from build123d import *

# Parameters (mm, degrees)
SKETCH_1_R      = 13
SKETCH_1_R_2    = 2
SKETCH_1_R_3    = 1.5
EXTRUDE_1_DEPTH = 3
FILLET_1_R      = 2


with BuildPart() as part:
    # 草图1 → 凸台-拉伸1 (new body)
    with BuildSketch(Plane.XY):
        with BuildLine():
            Line((0, 21), (32.5, 21))
            Line((32.5, 21), (32.5, 5))
            Line((32.5, 5), (47.5, 5))
            Line((47.5, 5), (47.5, 8))
            ThreePointArc((47.5, 8), (49, 9.5), (50.5, 8))
            Line((50.5, 8), (50.5, -21))
            Line((50.5, -21), (0, -21))
            ThreePointArc((0, -21), (-21, 0), (0, 21))
        make_face()
        Circle(SKETCH_1_R, mode=Mode.SUBTRACT)
        with Locations((17.5, 0)):
            Circle(SKETCH_1_R_2, mode=Mode.SUBTRACT)
        with Locations((0, -17.5)):
            Circle(SKETCH_1_R_2, mode=Mode.SUBTRACT)
        with Locations((-17.5, 0)):
            Circle(SKETCH_1_R_2, mode=Mode.SUBTRACT)
        with Locations((0, 17.5)):
            Circle(SKETCH_1_R_2, mode=Mode.SUBTRACT)
        with Locations((40, -7.5)):
            Circle(SKETCH_1_R_3, mode=Mode.SUBTRACT)
        with Locations((40, -17.5)):
            Circle(SKETCH_1_R_3, mode=Mode.SUBTRACT)
        with Locations((24.5, 15)):
            Circle(SKETCH_1_R_3, mode=Mode.SUBTRACT)
        with Locations((24.5, -15)):
            Circle(SKETCH_1_R_3, mode=Mode.SUBTRACT)
    extrude(amount=EXTRUDE_1_DEPTH)

    # 圆角1
    fillet_1_edges = [part.edges().sort_by_distance(p)[0] for p in [
        (32.5, 21, 1.5),
        (50.5, -21, 1.5),
    ]]
    fillet(fillet_1_edges, radius=FILLET_1_R)


solid = part.part
Input: part model. Units: mm. Frame: model coordinates. A direction names the side the tool comes from. Coordinates: 2 decimals unless noted, no trailing zeros. Loops run counter-clockwise (first coordinate to the right, second up) from the corner with the lowest first, then second, coordinate; pieces in that order, holes last. Notation, with made-up numbers: (85, 29) -> (144, 29) arc R16 ccw to (144, 36) -> close; hole circle Ø1 at (59.5, -18.75). An arc over 180 degrees is marked (long way). Write each question's results on one line, items separated by ' | '. Start each with the question number.
Q1. Section D-D, the plane x = -6. Return the cut outline in (y, z), plus the area to 3 significant figures.
Q2. Section C-C, the plane y = 11. Return the cut outline in (x, z).
Q3. Section B-B, the plane z = 2.5. State how many separate pieces and enclosed holes the cut face has, plus the area to 3 significant figures.
Q4. Reachability of faces 1 (the flat face through (32.5, 12, 1)), 2 (the flat face through (50.5, -5, 1)) from +Z, -Z, +X, -X, +Y, -Y: full face, straight path, thin tool, end or side. Return the list, or none.
Q5. Pin query (flat end, axial travel): pin 1 (0.9 mm diameter, centred on x = 40.5, z = 2, fed in from +Y); pin 2 (3 mm diameter, centred on x = 0, y = 17.5, fed in from +Z); pin 3 (1 mm diameter, centred on x = -8, z = 0.5, fed in from -Y). Return the tip coordinate at first contact, or that it passes through.
Q6. Section A-A, the plane x = 40. Return the cut outline in (y, z).
Q7. Ray query, line 1 (Y direction, x = 24.5, z = 1.6); line 2 (X direction, y = -18, z = 1.8); line 3 (X direction, y = 7, z = 0.6). Return the intervals inside material, ascending. Write a range as from..to.
Q8. Pull-direction query (Y, two-part tool) for faces 3 (the flat face through (40, 5, 1)), 4 (the flat face through (23, 0, 0)), 5 (the cylindrical face through (-19.1, -1.2, 1.5)); classes: released by +Y, released by -Y, zero draft, split by the parting line, or undercut.
Found:
1) outline: (-20.12, 0) -> (-11.53, 0) -> (-11.53, 3) -> (-20.12, 3) -> close; (11.53, 0) -> (20.12, 0) -> (20.12, 3) -> (11.53, 3) -> close | area: 51.6 mm2
2) outline: (-17.89, 0) -> (-6.93, 0) -> (-6.93, 3) -> (-17.89, 3) -> close; (6.93, 0) -> (32.5, 0) -> (32.5, 3) -> (6.93, 3) -> close
3) separate pieces: 1 | enclosed holes: 9 | area: 1,930 mm2
4) face 1: +Z, -Z, +Y | face 2: +Z, -Z, +X, +Y, -Y
5) pin 1: y = 5 | pin 2: through | pin 3: y = -19.62
6) outline: (-21, 0) -> (-19, 0) -> (-19, 3) -> (-21, 3) -> close; (-16, 0) -> (-9, 0) -> (-9, 3) -> (-16, 3) -> close; (-6, 0) -> (5, 0) -> (5, 3) -> (-6, 3) -> close
7) line 1: -21..-16.5, -13.5..13.5, 16.5..21 | line 2: -10.82..-1.94, 1.94..38.59, 41.41..50.5 | line 3: -19.8..-10.95, 10.95..32.5, 47.5..50.5
8) face 3: released by +Y | face 4: zero draft | face 5: undercut
